Source: CAD feature listing. Evaluate the final solid. Frame: model axes, mm. A direction names the side the tool comes from. Coordinates: 2 decimals unless noted, no trailing zeros. Order: outer loops, then holes, each group sorted by start corner. A loop starts at its lowest first (then second) coordinate and runs counter-clockwise, first axis right, second up.
Item 1: Reachability of faces 4 (the flat face through (-9.918, -4.785, -15.859)), 5 (the flat face through (15.671, -4.785, 9.542)), 6 (the flat face through (-15.9, -1.61, 9.9)), 7 (the flat face through (-9.542, -1.565, 15.671)) from +Z, -Z, +X, -X, +Y, -Y: full face, straight path, thin tool, end or side. Return the list, or none.
Item 2: Section C-C on y = -1.75. Return the cut outline in (x, z), then the cut area to 3 significant figures.
Item 3: Mould query, pull axis X, two halves, no side actions, for faces 1 (the flat face through (9.918, -4.785, 15.859)), 2 (the flat face through (0, 0, 0)), 3 (the flat face through (15.71, -1.61, 9.52)). Classes: released by +X, released by -X, zero draft, split by the parting line, or undercut.
Item 4: Contact query for flat-ended pins moving along their axis: P1, Ø3, axis at x = -2.5, y = -2, coming from the +Z side; P2, Ø1, axis at x = 5, y = -1.5, coming from the -Z side. Output: stop coordinate, or through.
Item 5: Ray query, line 1 (X direction, y = -6, z = -14); line 2 (Z direction, x = -17, y = -3.5); line 3 (X direction, y = -2, z = 16). Return the intervals inside material, ascending.
from build123d import *

# Parameters (mm, degrees)
F1_DEPTH = 6.35
F2_SIZE  = 3.175
F3_SIZE  = 3.17499


# Not quite as in the source:
# - a fillet or chamfer is up to 0.001 mm smaller than in the source, because OpenCascade refuses the exact size


with BuildPart() as f1:
    # F0 (on Front) → F1 (new body)
    with BuildSketch(Plane.XZ):
        Polygon((0, 12.7), (-25.4, 25.4), (-12.7, 0), (-25.4, -25.4), (0, -12.7), (25.4, -25.4), (12.7, 0), (25.4, 25.4), align=None)
    extrude(amount=F1_DEPTH)

    # F2
    f2_edges = [f1.edges().sort_by_distance(p)[0] for p in [
        (-19.05, -6.35, 12.7),
        (-12.7, -6.35, 19.05),
        (12.7, -6.35, -19.05),
        (19.05, -6.35, -12.7),
        (19.05, -6.35, 12.7),
        (12.7, -6.35, 19.05),
        (-19.05, -6.35, -12.7),
        (-12.7, -6.35, -19.05),
    ]]
    chamfer(f2_edges, length=F2_SIZE)

    # F3 (size 3.175 in the source; OpenCascade refuses exactly that, so slightly less here)
    f3_edges = [f1.edges().sort_by_distance(p)[0] for p in [
        (-19.05, 0, -12.7),
        (-12.7, 0, -19.05),
        (12.7, 0, -19.05),
        (19.05, 0, -12.7),
        (19.05, 0, 12.7),
        (12.7, 0, 19.05),
        (-12.7, 0, 19.05),
        (-19.05, 0, 12.7),
    ]]
    chamfer(f3_edges, length=F3_SIZE)


solid = f1.part
Answer list:
1. face 4: -Z, -Y
1. face 5: +X, -Y
1. face 6: -X, +Y
1. face 7: +Z, +Y
2. outline: (-22.21, -22.21) - (0, -11.11) - (22.21, -22.21) - (11.11, 0) - (22.21, 22.21) - (0, 11.11) - (-22.21, 22.21) - (-11.11, 0) - close
2. area: 987 mm2
3. face 1: undercut
3. face 2: zero draft
3. face 3: released by +X
4. P1: stops at z = 14.42
4. P2: stops at z = -13.94
5. line 1: x = -16.54 to -8.92, 8.92 to 16.54
5. line 2: z = -20.84 to -9.33, 9.33 to 20.84
5. line 3: x = -19.39 to -9.23, 9.23 to 19.39
